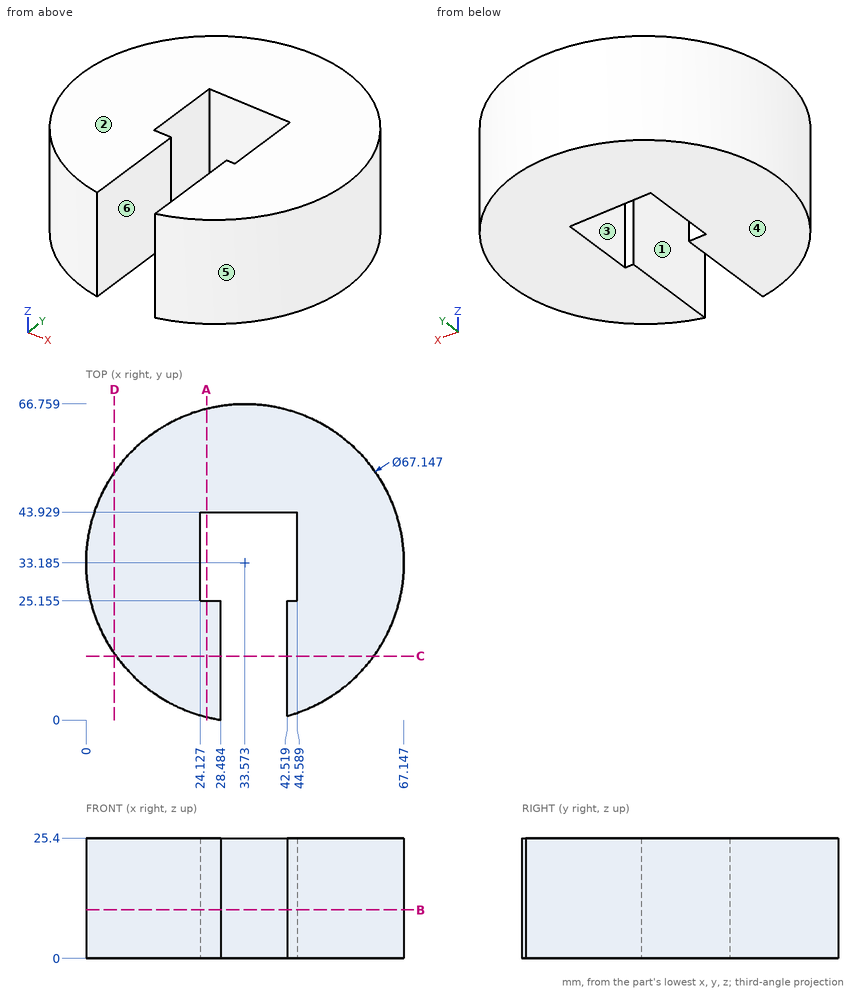
Geometry check sheet. Reference: drawing and pictorial views, mm from the part's lowest x, y, z. A direction names the side the tool comes from. Give positions to 0.01 mm unless a question says otherwise; leave off trailing zeros. Write each loop counter-clockwise with the first axis right and the second up, starting at its lowest first coordinate (ties: lowest second). Pieces come first, ordered by that corner, then holes. Notation, with made-up numbers: M 37.5,-26.75 L 46.5,-26.75 A6 ccw 46.5,-16.75 Z; hole C 23,-6.5 d9. An arc over 180 degrees is marked long. Answer as CSV lines item,"result". Start each with the question number.
Q1. Tool access check on the marked faces 1, 2 and 3. Record the directions out of +Z, -Z, +X, -X, +Y, -Y that give a thin tool (end or side, any length) a straight path to the whole face; none if there is none.
Q2. Material ranges on L1, parallel to X at y = 42, z = 21.5; L2, parallel to X at y = 28, z = 2.75 (1 decimal); L3, parallel to Y at x = 43, z = 17.5 (1 decimal), recorded low to high.
Q3. Section check A-A, the plane x = 25.5. Record the cut outline in (y, z) (1 decimal).
Q4. Section check D-D, the plane x = 6. Record the cut outline in (y, z).
Q5. Section check B-B, the plane z = 10.25. Record the cut outline in (x, y) (1 decimal).
Q6. Go/stop test with flat-tipped pins: pin 1 (3 mm diameter, centred on y = 54.5, z = 17.5, fed in from +X) (1 decimal); pin 2 (2 mm diameter, centred on y = 54.5, z = 4, fed in from -X) (1 decimal); pin 3 (2 mm diameter, centred on y = 16.5, z = 12.5, fed in from +X). Record where each tip stops, or that it passes through.
Q7. Release check for a two-part mould opening along X. For the marked faces 4, 5 and 6 record: pulls with the +X half, pulls with the -X half, needs draft (parallel to the pull), parting line crosses it, or undercut.
Q8. Section check C-C, the plane y = 13.5. Record the cut outline in (x, z), then the cut area to 4 significant figures.
Geometry says:
1,face 1,"+Z, -Z, -Y"
1,face 2,"+Z, +X, -X, +Y, -Y"
1,face 3,"+Z, -Z"
2,L1,"1.18 to 24.13, 44.59 to 65.97"
2,L2,"0.4 to 24.1, 44.6 to 66.7"
2,L3,"1 to 25.2, 43.9 to 65.4"
3,outline,"M 0.6,0 L 25.2,0 L 25.2,25.4 L 0.6,25.4 Z; M 43.9,0 L 65.8,0 L 65.8,25.4 L 43.9,25.4 Z"
4,outline,"M 14.03,0 L 52.34,0 L 52.34,25.4 L 14.03,25.4 Z"
5,outline,"M 24.1,25.2 L 24.1,43.9 L 44.6,43.9 L 44.6,25.2 L 42.5,25.2 L 42.5,0.8 A33.6 ccw long 28.5,0 L 28.5,25.2 Z"
6,pin 1,"x = 60.7"
6,pin 2,"x = 6.8"
6,pin 3,"x = 63.26"
7,face 4,"needs draft"
7,face 5,"parting line crosses it"
7,face 6,"undercut"
8,outline,"M 6.38,0 L 28.48,0 L 28.48,25.4 L 6.38,25.4 Z; M 42.52,0 L 60.77,0 L 60.77,25.4 L 42.52,25.4 Z"
8,area,"1,025 mm^2"
